The listing builds one solid part. Answer for the finished solid, in the listing's coordinates (mm). A direction names the side the tool comes from. Coordinates: 2 decimals unless noted, no trailing zeros. Order: outer loops, then holes, each group sorted by start corner. A loop starts at its lowest first (then second) coordinate and runs counter-clockwise, first axis right, second up. Notation, with made-up numbers: (11, 86) -> (67, 86) arc R21 ccw to (67, 112) -> close; hole circle Ø3 at (7, -38.5). An arc over 180 degrees is marked (long way). Return JSON: item names as keys, results as strings.
from build123d import *

# Parameters (mm, degrees)
SKETCH1_W           = 2.5
SKETCH1_H           = 25
BOSS_EXTRUDE3_DEPTH = 2
BOSS_EXTRUDE4_DEPTH = 12
FILLET2_R           = 4


with BuildPart() as part:
    # Sketch1 → Boss-Extrude3 (new body)
    with BuildSketch(Plane.XY):
        Polygon((19.027950311, 8.201863354), (-10.472049689, 8.201863354), (-7.972049689, 5.701863354), (-5.472049689, 5.701863354), (-2.972049689, 5.701863354), (-0.472049689, 5.701863354), (4.527950311, 5.701863354), (7.027950311, 5.701863354), (14.027950311, 5.701863354), (16.527950311, 5.701863354), (19.027950311, 5.701863354), align=None)
        Polygon((-7.972049689, -19.298136646), (-7.972049689, 5.701863354), (-10.472049689, 5.701863354), (-10.472049689, -21.798136646), align=None)
        Polygon((-7.972049689, 5.701863354), (-10.472049689, 8.201863354), (-10.472049689, 5.701863354), align=None)
        Polygon((-2.972049689, 5.701863354), (-5.472049689, 5.701863354), (-5.472049689, -19.298136646), (-7.972049689, -19.298136646), (-10.472049689, -21.798136646), (19.027950311, -21.798136646), (19.027950311, 5.701863354), (16.527950311, 5.701863354), (16.527950311, -19.298136646), (14.027950311, -19.298136646), (14.027950311, 5.701863354), (7.027950311, 5.701863354), (7.027950311, -19.298136646), (4.527950311, -19.298136646), (4.527950311, 5.701863354), (-0.472049689, 5.701863354), (-0.472049689, -19.298136646), (-2.972049689, -19.298136646), align=None)
        with Locations((5.777950311, -6.798136646)):
            Rectangle(SKETCH1_W, SKETCH1_H)
        with Locations((15.277950311, -6.798136646)):
            Rectangle(SKETCH1_W, SKETCH1_H)
        with Locations((-1.722049689, -6.798136646)):
            Rectangle(SKETCH1_W, SKETCH1_H)
        with Locations((-6.722049689, -6.798136646)):
            Rectangle(SKETCH1_W, SKETCH1_H)
    extrude(amount=BOSS_EXTRUDE3_DEPTH)

    # Sketch1_8 → Boss-Extrude4 (add)
    with BuildSketch(Plane.XY):
        Polygon((-2.972049689, 5.701863354), (-5.472049689, 5.701863354), (-5.472049689, -19.298136646), (-7.972049689, -19.298136646), (-10.472049689, -21.798136646), (19.027950311, -21.798136646), (19.027950311, 5.701863354), (16.527950311, 5.701863354), (16.527950311, -19.298136646), (14.027950311, -19.298136646), (14.027950311, 5.701863354), (7.027950311, 5.701863354), (7.027950311, -19.298136646), (4.527950311, -19.298136646), (4.527950311, 5.701863354), (-0.472049689, 5.701863354), (-0.472049689, -19.298136646), (-2.972049689, -19.298136646), align=None)
        Polygon((19.027950311, 8.201863354), (-10.472049689, 8.201863354), (-7.972049689, 5.701863354), (-5.472049689, 5.701863354), (-2.972049689, 5.701863354), (-0.472049689, 5.701863354), (4.527950311, 5.701863354), (7.027950311, 5.701863354), (14.027950311, 5.701863354), (16.527950311, 5.701863354), (19.027950311, 5.701863354), align=None)
        Polygon((-7.972049689, -19.298136646), (-7.972049689, 5.701863354), (-10.472049689, 5.701863354), (-10.472049689, -21.798136646), align=None)
        Polygon((-7.972049689, 5.701863354), (-10.472049689, 8.201863354), (-10.472049689, 5.701863354), align=None)
    extrude(amount=BOSS_EXTRUDE4_DEPTH)

    # Fillet2
    fillet2_edges = [part.edges().sort_by_distance(p)[0] for p in [
        (-10.472049689, 8.201863354, 6),
        (19.027950311, 8.201863354, 6),
        (19.027950311, -21.798136646, 6),
        (-10.472049689, -21.798136646, 6),
    ]]
    fillet(fillet2_edges, radius=FILLET2_R)


solid = part.part
1. This flat-tipped pin is pushed along its axis until it touches: pin 1 Ø1.5 at (x, y) = (-6.5, -17.5) entering from +Z. Where does it stop, or does it pass through?
Answer block:
{"pin 1": "stops at z = 2"}
2. The part is cut by section B-B on x = 14.5. Give the vertices of the cut face in (y, z), and give its area (3 significant figures).
Answer block:
{"outline": "(-21.8, 0) -> (8.2, 0) -> (8.2, 12) -> (5.7, 12) -> (5.7, 2) -> (-19.3, 2) -> (-19.3, 12) -> (-21.8, 12) -> close", "area": "110 mm2"}
3. The part is cut by section C-C on y = -5. Give the vertices of the cut face in (x, z).
Answer block:
{"outline": "(-10.47, 0) -> (19.03, 0) -> (19.03, 12) -> (16.53, 12) -> (16.53, 2) -> (14.03, 2) -> (14.03, 12) -> (7.03, 12) -> (7.03, 2) -> (4.53, 2) -> (4.53, 12) -> (-0.47, 12) -> (-0.47, 2) -> (-2.97, 2) -> (-2.97, 12) -> (-5.47, 12) -> (-5.47, 2) -> (-7.97, 2) -> (-7.97, 12) -> (-10.47, 12) -> close"}
4. Determine the mould class of faces 3 (the face through (19.028, -7, 6)), 4 (the face through (-7, 5.702, 7)), 5 (the face through (-9.269, -20.657, 6.084)) for opening direction Y: pulls with the +Y half, pulls with the -Y half, needs draft (parallel to the pull), parting line crosses it, or undercut.
Answer block:
{"face 3": "needs draft", "face 4": "undercut", "face 5": "pulls with the -Y half"}
5. The part is cut by section A-A on z = 9.25. Give the vertices of the cut face in (x, y).
Answer block:
{"outline": "(-10.47, -17.8) arc R4 ccw to (-6.47, -21.8) -> (15.03, -21.8) arc R4 ccw to (19.03, -17.8) -> (19.03, 4.2) arc R4 ccw to (15.03, 8.2) -> (-6.47, 8.2) arc R4 ccw to (-10.47, 4.2) -> close; hole (-7.97, -19.3) -> (-5.47, -19.3) -> (-5.47, 5.7) -> (-7.97, 5.7) -> close; hole (-2.97, -19.3) -> (-0.47, -19.3) -> (-0.47, 5.7) -> (-2.97, 5.7) -> close; hole (4.53, -19.3) -> (7.03, -19.3) -> (7.03, 5.7) -> (4.53, 5.7) -> close; hole (14.03, -19.3) -> (16.53, -19.3) -> (16.53, 5.7) -> (14.03, 5.7) -> close"}
6. Consider line 1 (X direction, y = -14.75, z = 9.75); line 2 (Y direction, x = 5.5, z = 7); line 3 (X direction, y = -18.25, z = 3.5). Determine where each line is inside the solid, lowest interval first. Write a range as from..to.
Answer block:
{"line 1": "x = -10.47..-7.97, -5.47..-2.97, -0.47..4.53, 7.03..14.03, 16.53..19.03", "line 2": "y = -21.8..-19.3, 5.7..8.2", "line 3": "x = -10.45..-7.97, -5.47..-2.97, -0.47..4.53, 7.03..14.03, 16.53..19"}
7. The part is cut by section D-D on z = 1. Give the vertices of the cut face in (x, y).
Answer block:
{"outline": "(-10.47, -17.8) arc R4 ccw to (-6.47, -21.8) -> (15.03, -21.8) arc R4 ccw to (19.03, -17.8) -> (19.03, 4.2) arc R4 ccw to (15.03, 8.2) -> (-6.47, 8.2) arc R4 ccw to (-10.47, 4.2) -> close"}
8. For faces 1 (the face through (4, 8.202, 6)), 2 (the face through (-7.972, -7, 7)), determine the directions among +Z, -Z, +X, -X, +Y, -Y from which every point of the face is accessible in a straight line to the end or side of a thin tool.
Answer block:
{"face 1": "+Z, -Z, +X, -X, +Y", "face 2": "+Z"}
